Could you check a few things on this model? Use its own coordinates, in mm. A direction names the side the tool comes from. Give positions to 0.01 mm unless a question says otherwise; leave off trailing zeros. Loops run counter-clockwise (first coordinate to the right, second up) from the corner with the lowest first, then second, coordinate; pieces in that order, holes last. Notation, with made-up numbers: M 78.5,-21 L 105.5,-21 A5 ccw 105.5,-14 Z; hole C -28,-5.75 d11. An arc over 180 degrees is marked long. Use a Markdown table: item, result. Add a question column.
1) Will these pins go through, and if not, where does the flat tip stop? pin 1 Ø3 at (x, z) = (0, 0) entering from -Y; pin 2 Ø3 at (x, z) = (-1, -0.5) entering from +Y; pin 3 Ø2 at (x, y) = (-1.5, 5) entering from -Z.
2) Suppose I cut it at A-A on y = 9.25. List the corners of the cut face in (x, z) for me, and give its area (3 significant figures).
3) Suppose I cut it at B-B on y = 1.75. List the corners of the cut face in (x, z) for me.
4) We'd pull the mould along X, two halves only. Please class faces 1 (the cylindrical face through (-0.596, 7.2, 2.685)), 2 (the flat face through (0, 0.1, 0)), 3 (the flat face through (-1, 12, 2)): +X half, -X half, draft (parallel to the pull), parting line (faces both ways), or undercut.
5) If I drill on line 1 along Y through (x, z) = (-1.5, -0.6); line 2 along Z through (x, y) = (-1.3, 1.5); line 3 along X through (y, z) = (6, -1.3), over which ranges is the centre line in solid material (lowest first)? Write a range as [from, to].
6) Which directions (+Z, -Z, +X, -X, +Y, -Y) give clear straight access to the entire face, cutting with the end or side of a thin tool? Please do faces 4 (the flat face through (-1, 0, 2)), 5 (the flat face through (0, 11.9, 0)).
```python
from build123d import *

# Parameters (mm, degrees)
SKETCH1_R           = 2.75
BOSS_EXTRUDE1_DEPTH = 12
FILLET2_R           = 0.3
FILLET3_R           = 0.3
FILLET4_R           = 0.7
SKETCH3_R           = 2
CUT_EXTRUDE1_DEPTH  = 0.1
SKETCH5_R           = 2
CUT_EXTRUDE3_DEPTH  = 0.1


with BuildPart() as part:
    # Sketch1 → Boss-Extrude1 (new body)
    with BuildSketch(Plane(origin=(0, 0, 0), x_dir=(1, 0, 0), z_dir=(0, 1, 0))):
        Circle(SKETCH1_R)
    extrude(amount=BOSS_EXTRUDE1_DEPTH)

    # Sketch2 → Cut-Revolve1 (revolve, cut)
    with BuildSketch(Plane.XY):
        with BuildLine():
            Line((2.75, 2.67418437), (2.75, 1.507628734))
            ThreePointArc((2.75, 1.507628734), (2.609122054, 2.090906552), (2.75, 2.67418437))
        make_face()
    revolve(axis=Axis((0, 0, 0), (0, 1, 0)), mode=Mode.SUBTRACT)

    # Fillet2
    fillet2_edges = [part.edges().sort_by_distance(p)[0] for p in [
        (-2.75, 12, 0),
    ]]
    fillet(fillet2_edges, radius=FILLET2_R)

    # Fillet3
    fillet3_edges = [part.edges().sort_by_distance(p)[0] for p in [
        (-2.75, 0, 0),
    ]]
    fillet(fillet3_edges, radius=FILLET3_R)

    # Fillet4
    fillet4_edges = [part.edges().sort_by_distance(p)[0] for p in [
        (-2.75, 1.507628734, 0),
        (-2.75, 2.67418437, 0),
    ]]
    fillet(fillet4_edges, radius=FILLET4_R)

    # Sketch3 → Cut-Extrude1 (cut)
    with BuildSketch(Plane(origin=(0, 12, 0), x_dir=(1, 0, 0), z_dir=(0, 1, 0))):
        Circle(SKETCH3_R)
    extrude(amount=-CUT_EXTRUDE1_DEPTH, mode=Mode.SUBTRACT)

    # Sketch5 → Cut-Extrude3 (cut)
    with BuildSketch(Plane.XZ):
        Circle(SKETCH5_R)
    extrude(amount=-CUT_EXTRUDE3_DEPTH, mode=Mode.SUBTRACT)


solid = part.part
```
Answer block:
| question | item | result |
|---|---|---|
| 1 | pin 1 | stops at y = 0.1 |
| 1 | pin 2 | stops at y = 12 |
| 1 | pin 3 | stops at z = -2.7 |
| 2 | outline | C 0,0 d5.5 |
| 2 | area | 23.8 mm^2 |
| 3 | outline | C 0,0 d5.31 |
| 4 | face 1 | parting line |
| 4 | face 2 | undercut |
| 4 | face 3 | draft |
| 5 | line 1 | y = [0.1, 11.9] |
| 5 | line 2 | z = [-2.41, 2.41] |
| 5 | line 3 | x = [-2.42, 2.42] |
| 6 | face 4 | +Z, -Z, +X, -X, -Y |
| 6 | face 5 | +Y |
